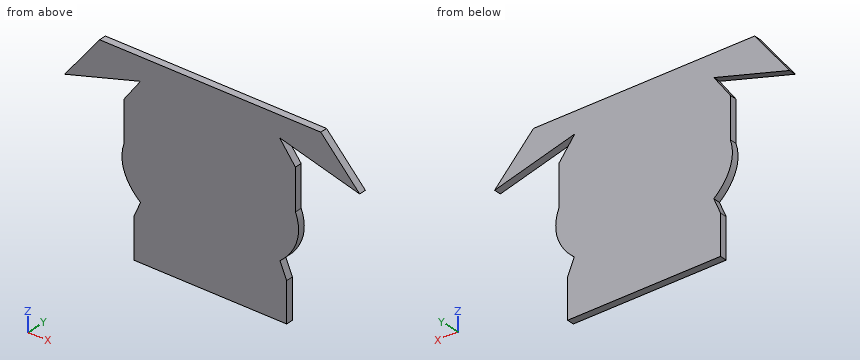
```python
from build123d import *

# Parameters (mm, degrees)
F0_W     = 22.0716209825
F0_H     = 11.3639943302
F0_W_2   = 22.1128826787
F1_DEPTH = 3.175


with BuildPart() as f1:
    # F0 (on Front) → F1 (new body)
    with BuildSketch(Plane.XZ):
        with BuildLine():
            add(Edge.make_bspline(
                [(0, 77.2495130793), (-13.2024395854, 77.2495130793), (-23.7188442589, 72.0280801734)],
                knots=[1.5707963268, 1.5707963268, 1.5707963268, 2.2200254143, 2.2200254143, 2.2200254143], degree=2, weights=[1, 0.9477737356, 1]))
            ThreePointArc((0, 77.2495130793), (-14.9655593265, 88.7487135304), (-23.7188442589, 72.0280801734))
        make_face()
        with BuildLine():
            add(Edge.make_bspline(
                [(37.8281886895, 58.3899668587), (34.3045126324, 66.7722575902), (23.7188442589, 72.0280801734)],
                knots=[0.2683589556, 0.2683589556, 0.2683589556, 0.9215672393, 0.9215672393, 0.9215672393], degree=2, weights=[1, 0.9471372908, 1]))
            add(Edge.make_bspline(
                [(23.7188442589, 72.0280801734), (13.2024395854, 77.2495130793), (0, 77.2495130793)],
                knots=[0.9215672393, 0.9215672393, 0.9215672393, 1.5707963268, 1.5707963268, 1.5707963268], degree=2, weights=[1, 0.9477737356, 1]))
            add(Edge.make_bspline(
                [(0, 77.2495130793), (-13.2024395854, 77.2495130793), (-23.7188442589, 72.0280801734)],
                knots=[1.5707963268, 1.5707963268, 1.5707963268, 2.2200254143, 2.2200254143, 2.2200254143], degree=2, weights=[1, 0.9477737356, 1]))
            add(Edge.make_bspline(
                [(-23.7188442589, 72.0280801734), (-35.179956424, 66.3375965856), (-38.2993388492, 57.1490477352)],
                knots=[2.2200254143, 2.2200254143, 2.2200254143, 2.9230595545, 2.9230595545, 2.9230595545], degree=2, weights=[1, 0.9388514321, 1]))
            add(Edge.make_bspline(
                [(-38.2993388492, 57.1490477352), (-42.2983339169, 45.3694848208), (-30.9822451126, 35.8404089541)],
                knots=[2.9230595545, 2.9230595545, 2.9230595545, 3.8020524721, 3.8020524721, 3.8020524721], degree=2, weights=[1, 0.9049660266, 1]))
            Line((-30.9822451126, 35.8404089541), (-33.9723048082, 28.8538616849))
            Line((-33.9723048082, 28.8538616849), (-33.9723048082, 22.5029981736))
            Line((-33.9723048082, 22.5029981736), (-11.8594221295, 22.5029981736))
            Line((-11.8594221295, 22.5029981736), (-11.8594221295, 11.1390038435))
            Line((-11.8594221295, 11.1390038435), (11.8594221295, 11.1390038435))
            Line((11.8594221295, 11.1390038435), (11.8594221295, 22.5029981736))
            Line((11.8594221295, 22.5029981736), (33.931043112, 22.5029981736))
            Line((33.931043112, 22.5029981736), (33.931043112, 28.8538616849))
            Line((33.931043112, 28.8538616849), (30.9822451126, 35.8404089541))
            add(Edge.make_bspline(
                [(30.9822451126, 35.8404089541), (43.0393262584, 45.9934612106), (37.8281886895, 58.3899668587)],
                knots=[5.6227254887, 5.6227254887, 5.6227254887, 6.5515442627, 6.5515442627, 6.5515442627], degree=2, weights=[1, 0.894086254, 1]))
        make_face()
        with BuildLine():
            add(Edge.make_bspline(
                [(23.7188442589, 57.1490477352), (23.7188442589, 89.4658166317), (-16.7717556174, 66.614410199), (-57.2623554937, 43.7630037663), (0, 43.7630037663)],
                knots=[0, 0, 0, 2.3561944902, 2.3561944902, 4.7123889804, 4.7123889804, 4.7123889804], degree=2, weights=[1, 0.3826834324, 1, 0.3826834324, 1]))
            add(Edge.make_bspline(
                [(0, 43.7630037663), (23.7188442589, 43.7630037663), (23.7188442589, 57.1490477352)],
                knots=[4.7123889804, 4.7123889804, 4.7123889804, 6.2831853072, 6.2831853072, 6.2831853072], degree=2, weights=[1, 0.7071067812, 1]))
        make_face(mode=Mode.SUBTRACT)
        with Locations((22.8952326207, 16.8210010086)):
            Rectangle(F0_W, F0_H)
        with BuildLine():
            add(Edge.make_bspline(
                [(23.7188442589, 72.0280801734), (13.2024395854, 77.2495130793), (0, 77.2495130793)],
                knots=[0.9215672393, 0.9215672393, 0.9215672393, 1.5707963268, 1.5707963268, 1.5707963268], degree=2, weights=[1, 0.9477737356, 1]))
            ThreePointArc((23.7188442589, 72.0280801734), (14.8063132284, 88.0253233293), (0, 77.2495130793))
        make_face()
        with BuildLine():
            add(Edge.make_bspline(
                [(0, 43.7630037663), (23.7188442589, 43.7630037663), (23.7188442589, 57.1490477352)],
                knots=[4.7123889804, 4.7123889804, 4.7123889804, 6.2831853072, 6.2831853072, 6.2831853072], degree=2, weights=[1, 0.7071067812, 1]))
            add(Edge.make_bspline(
                [(23.7188442589, 57.1490477352), (23.7188442589, 89.4658166317), (-16.7717556174, 66.614410199), (-57.2623554937, 43.7630037663), (0, 43.7630037663)],
                knots=[0, 0, 0, 2.3561944902, 2.3561944902, 4.7123889804, 4.7123889804, 4.7123889804], degree=2, weights=[1, 0.3826834324, 1, 0.3826834324, 1]))
        make_face()
        with BuildLine():
            ThreePointArc((0, 77.2495130793), (14.8063132284, 88.0253233293), (23.7188442589, 72.0280801734))
            add(Edge.make_bspline(
                [(37.8281886895, 58.3899668587), (34.3045126324, 66.7722575902), (23.7188442589, 72.0280801734)],
                knots=[0.2683589556, 0.2683589556, 0.2683589556, 0.9215672393, 0.9215672393, 0.9215672393], degree=2, weights=[1, 0.9471372908, 1]))
            Line((37.8281886895, 58.3899668587), (37.8281886895, 76.7098173911))
            Line((37.8281886895, 76.7098173911), (30.7735164742, 86.026978908))
            Line((30.7735164742, 86.026978908), (66.3792615504, 76.7098173911))
            Line((66.3792615504, 76.7098173911), (49.1188442589, 95.3441404248))
            Line((49.1188442589, 95.3441404248), (23.7188442589, 95.3441404248))
            Line((23.7188442589, 95.3441404248), (-23.7188442589, 95.3441404248))
            Line((-23.7188442589, 95.3441404248), (-49.1188442589, 95.3441404248))
            Line((-49.1188442589, 95.3441404248), (-64.6933734609, 75.2793942231))
            Line((-64.6933734609, 75.2793942231), (-31.0090915541, 85.311767324))
            Line((-31.0090915541, 85.311767324), (-38.2993388492, 75.2793942231))
            Line((-38.2993388492, 75.2793942231), (-38.2993388492, 57.1490477352))
            add(Edge.make_bspline(
                [(-23.7188442589, 72.0280801734), (-35.179956424, 66.3375965856), (-38.2993388492, 57.1490477352)],
                knots=[2.2200254143, 2.2200254143, 2.2200254143, 2.9230595545, 2.9230595545, 2.9230595545], degree=2, weights=[1, 0.9388514321, 1]))
            ThreePointArc((-23.7188442589, 72.0280801734), (-14.9655593265, 88.7487135304), (0, 77.2495130793))
        make_face()
        with Locations((-22.9158634688, 16.8210010086)):
            Rectangle(F0_W_2, F0_H)
    extrude(amount=-F1_DEPTH)


solid = f1.part
```
Build history of the part. All positions in model axes, mm. Give positions to 0.01 mm unless a question says otherwise; leave off trailing zeros. Loops run counter-clockwise (first coordinate to the right, second up) from the corner with the lowest first, then second, coordinate; pieces in that order, holes last. Notation, with made-up numbers: (48, -3.5) - (61, -3.5) arc R20 cw to (61, 24.5) - close; hole circle Ø2 at (80, 18.5). An arc over 180 degrees is marked (long way). Use a Markdown table: item, result.
(1) Drop a flat-ended pin along its axis: pin 1 Ø1 at (y, z) = (2, 66) entering from -X. Give the stop position or say it passes through.
Taken from the geometry:
| item | result |
|---|---|
| pin 1 | x = -38.3 |
(2) Band-saw the part on B-B (x = -47). Give the cut face in (y, z) (3 decimals), and give its area (3 significant figures).
Taken from the geometry:
| item | result |
|---|---|
| outline | (0, 80.549) - (3.175, 80.549) - (3.175, 95.344) - (0, 95.344) - close |
| area | 47.0 mm2 |
(3) Wall check: line 1 along Z through (x, y) = (33.5, 2.5); line 2 along Z through (x, y) = (-32.5, 0.65); line 3 along X through (y, z) = (2, 23.5). Give the ranges that are in metal, low to high.
Taken from the geometry:
| item | result |
|---|---|
| line 1 | 11.14 to 29.88, 38.23 to 82.43, 85.31 to 95.34 |
| line 2 | 11.14 to 32.29, 37.21 to 83.26, 84.87 to 95.34 |
| line 3 | -33.97 to 33.93 |
(4) Band-saw the part on A-A (z = 65). Give the cut face in (x, y) (3 decimals).
Taken from the geometry:
| item | result |
|---|---|
| outline | (-38.299, 0) - (37.828, 0) - (37.828, 3.175) - (-38.299, 3.175) - close |
